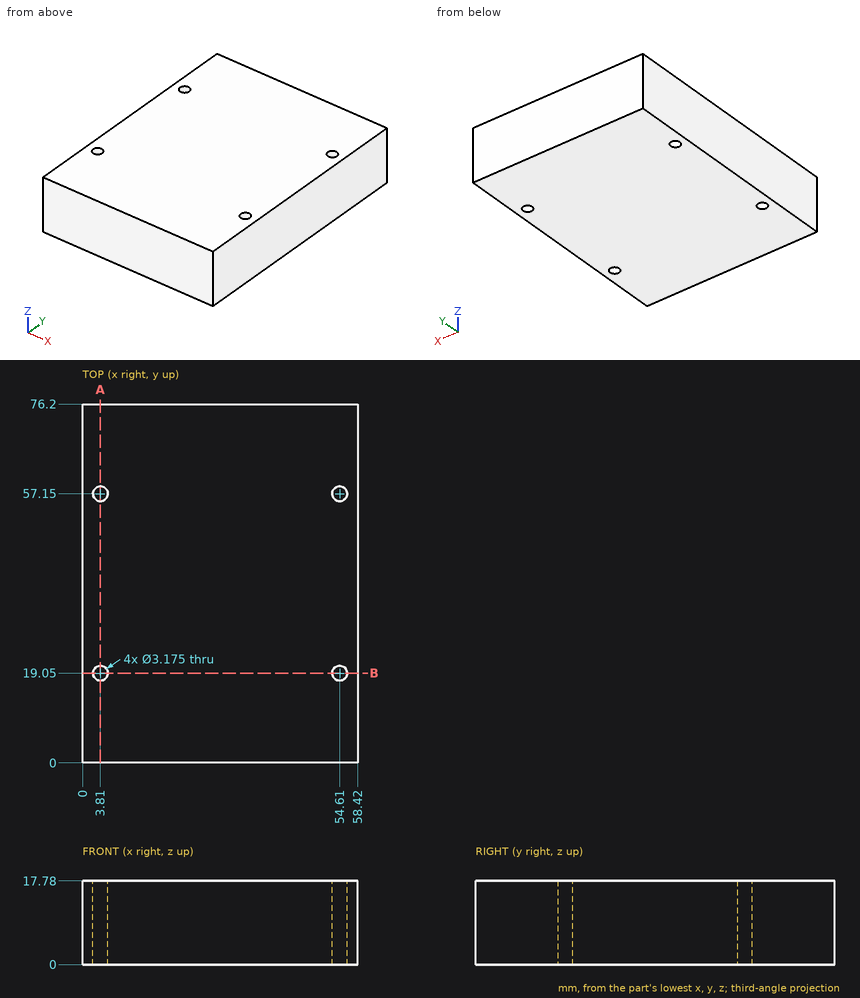
Drawing for the job (mm, zero at the part's lowest x, y, z). Coordinates: 2 decimals unless noted, no trailing zeros. Order: outer loops, then holes, each group sorted by start corner. A loop starts at its lowest first (then second) coordinate and runs counter-clockwise, first axis right, second up. Notation, with made-up numbers: (19.25, 80) - (26.25, 80) arc R35 cw to (26.25, 113) - close; hole circle Ø11 at (74, 2.5). An arc over 180 degrees is marked (long way). Use a Markdown table: item, result. Add a question column.
(1) Saw through at B-B (y = 19.05). Give the cut face in (x, z).
(2) Flat gauge pin, fed straight in: pin 1 (2.5 mm diameter, centred on x = 54.61, y = 57.15, fed in from +Z). Where does the tip first touch, or does it go through?
(3) Drill centre lines: line 1 along X through (y, z) = (57.15, 8.25); line 2 along Y through (x, z) = (54.5, 16.25); line 3 along X through (y, z) = (18.5, 6). Where is each one in solid material? Low to high. Write a range as [from, to].
(4) Saw through at A-A (x = 3.81). Give the cut face in (y, z).
Solved:
| question | item | result |
|---|---|---|
| 1 | outline | (0, 0) - (2.22, 0) - (2.22, 17.78) - (0, 17.78) - close; (5.4, 0) - (53.02, 0) - (53.02, 17.78) - (5.4, 17.78) - close; (56.2, 0) - (58.42, 0) - (58.42, 17.78) - (56.2, 17.78) - close |
| 2 | pin 1 | passes through |
| 3 | line 1 | x = [0, 2.22], [5.4, 53.02], [56.2, 58.42] |
| 3 | line 2 | y = [0, 17.47], [20.63, 55.57], [58.73, 76.2] |
| 3 | line 3 | x = [0, 2.32], [5.3, 53.12], [56.1, 58.42] |
| 4 | outline | (0, 0) - (17.46, 0) - (17.46, 17.78) - (0, 17.78) - close; (20.64, 0) - (55.56, 0) - (55.56, 17.78) - (20.64, 17.78) - close; (58.74, 0) - (76.2, 0) - (76.2, 17.78) - (58.74, 17.78) - close |
